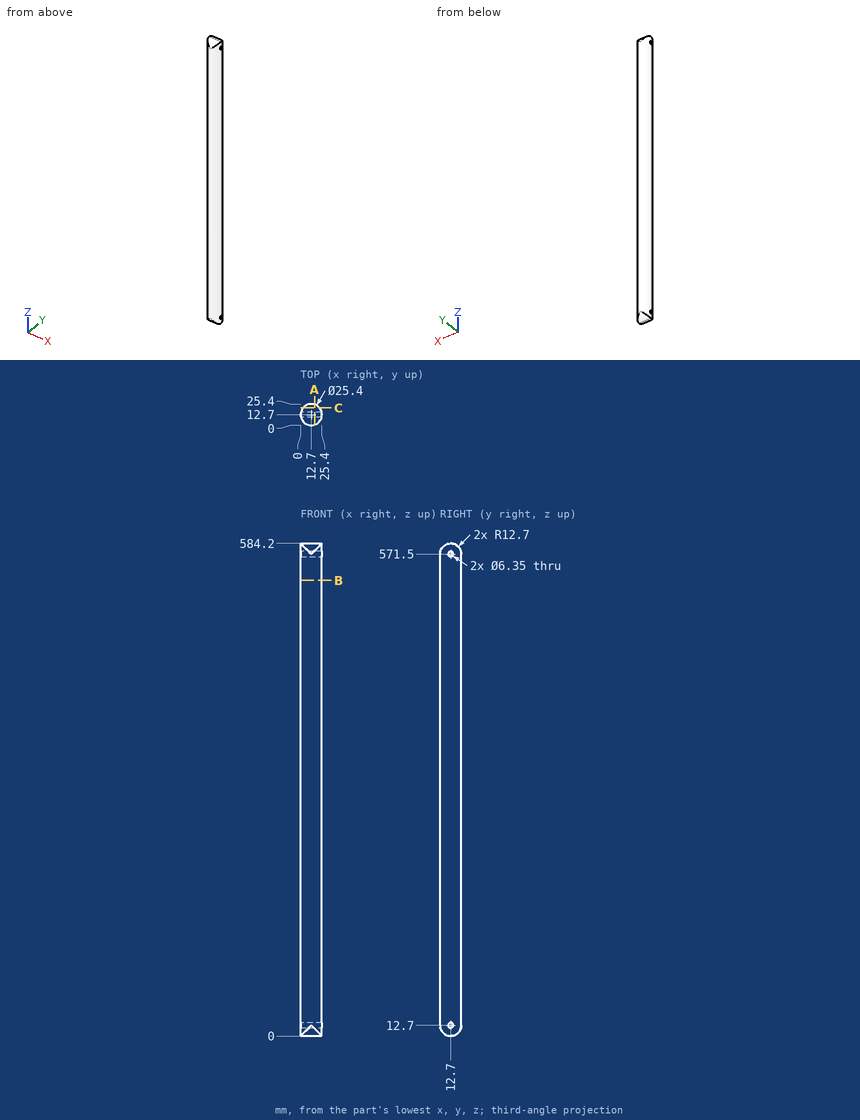
Study the drawing (mm; zero at the part's minimum x, y, z) and answer. Round coordinates to 2 decimals unless told otherwise and drop trailing zeros. Write each loop counter-clockwise with the first axis right and the second up, starting at its lowest first coordinate (ties: lowest second). Pieces come first, ordered by that corner, then holes.
1) A cutting plane is placed at A-A on x = 16.75. Determine the outline of the cut face in (y, z) (3 decimals).
2) Flat-ended cylindrical pins translate along their axes: P1, Ø4, axis at x = 16, y = 3.5, coming from the -Z side; P2, Ø10, axis at y = 3.5, z = 140, coming from the +X side; P3, Ø8, axis at x = 21.5, y = 5, coming from the -Z side. Find the tip coordinate at first contact, or state that the pin passes through.
3) A cutting plane is placed at C-C on y = 20.75. Determine the outline of the cut face in (x, z), and give its area (3 significant figures).
4) Consider probe 1 along Z at (x, y) = (12, 13); probe 2 along Y at (x, z) = (14.25, 571.5) (3 decimals); probe 3 along Z at (x, y) = (3.5, 11.25). Determine where each line is inside the solid, lowest interval first.
5) A cutting plane is placed at B-B on z = 540.5. Determine the outline of the cut face in (x, y), and give its area (3 significant figures).
Entries:
1. outline: (0.663, 8.65) arc R12.7 ccw to (24.737, 8.65) - (24.737, 575.55) arc R12.7 ccw to (0.663, 575.55) - close; hole circle Ø6.35 at (12.7, 12.7); hole circle Ø6.35 at (12.7, 571.5)
2. P1: stops at z = 2.24
2. P2: stops at x = 24.69
2. P3: stops at z = 0.55
3. outline: (2.88, 2.88) - (22.52, 2.88) - (22.52, 581.32) - (2.88, 581.32) - close
3. area: 11,400 mm2
4. probe 1: z = 0 to 9.54, 15.86 to 568.34, 574.66 to 584.2
4. probe 2: y = 0.095 to 9.525, 15.875 to 25.305
4. probe 3: z = 0.08 to 9.88, 15.52 to 568.68, 574.32 to 584.12
5. outline: circle Ø25.4 at (12.7, 12.7)
5. area: 507 mm2
